from build123d import *

# Parameters (mm, degrees)
BOSS_EXTRU_1_DEPTH = 15


with BuildPart() as part:
    # Esquisse1 → Boss.-Extru.1 (new body)
    with BuildSketch(Plane.XY):
        with BuildLine():
            ThreePointArc((-50, -27.5), (-47.071067812, -34.571067812), (-40, -37.5))
            Line((-40, -37.5), (-35, -37.5))
            Line((-35, -37.5), (-35, -22.5))
            Line((-35, -22.5), (-35, -7.5))
            Line((-35, -7.5), (-25, -7.5))
            Line((-25, -7.5), (-25, -22.5))
            Line((-25, -22.5), (25, -22.5))
            Line((25, -22.5), (25, -7.5))
            Line((25, -7.5), (35, -7.5))
            Line((35, -7.5), (35, -22.5))
            Line((35, -22.5), (35, -37.5))
            Line((35, -37.5), (40, -37.5))
            ThreePointArc((40, -37.5), (47.071067812, -34.571067812), (50, -27.5))
            Line((50, -27.5), (50, 27.5))
            ThreePointArc((50, 27.5), (47.071067812, 34.571067812), (40, 37.5))
            Line((40, 37.5), (7.5, 37.5))
            Line((7.5, 37.5), (7.5, 15))
            Line((7.5, 15), (-7.5, 15))
            Line((-7.5, 15), (-7.5, 37.5))
            Line((-7.5, 37.5), (-40, 37.5))
            ThreePointArc((-40, 37.5), (-47.071067812, 34.571067812), (-50, 27.5))
            Line((-50, 27.5), (-50, -27.5))
        make_face()
    extrude(amount=BOSS_EXTRU_1_DEPTH)


solid = part.part
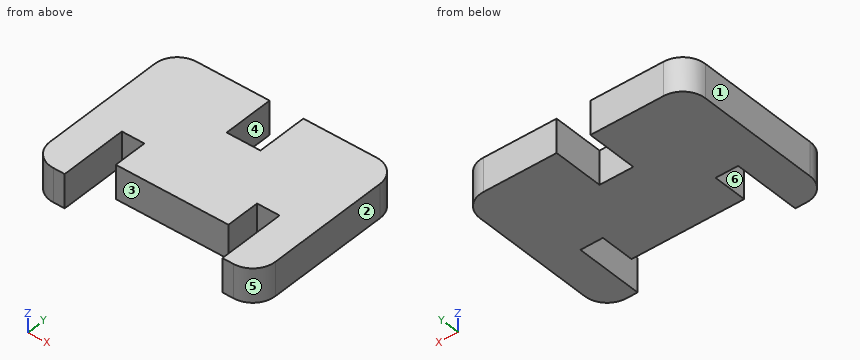
Check sheet for the modelled part. Datum: model origin and axes. Units: mm. Face numbers are marked on the shaded views. A direction names the side the tool comes from. Give positions to 0.01 mm unless a question says otherwise; leave off trailing zeros. Loops run counter-clockwise (first coordinate to the right, second up) from the corner with the lowest first, then second, coordinate; pieces in that order, holes last. Notation, with made-up numbers: M 56,24 L 83,24 A12 ccw 83,42 Z; hole C 47,70 d11. An arc over 180 degrees is marked long. Return JSON: item names as keys, results as strings. Group by question number.
1. Cross-section at D-D on y = -30. Record the boundary of the cut face in (x, z), plus the area to 3 significant figures.
2. Thickness scan on L1, parallel to X at y = -21, z = 3.25; L2, parallel to X at y = 20.5, z = 10.5; L3, parallel to X at y = -25.5, z = 4.75. Record the ranges inside material, lowest first.
3. Tool access check on the marked faces 4, 5 and 6. Record the directions out of +Z, -Z, +X, -X, +Y, -Y that give a thin tool (end or side, any length) a straight path to the whole face; none if there is none.
4. Cross-section at C-C on x = 6. Record the boundary of the cut face in (y, z), plus the area to 4 significant figures.
5. Cross-section at A-A on y = 17.5. Record the boundary of the cut face in (x, z).
6. Cross-section at B-B on z = 1.25. Record the boundary of the cut face in (x, y), plus the area to 3 significant figures.
7. Mould release check, pull along X, two halves, no side actions. Record for the marked faces 1, 2 and 3: released by +X, released by -X, zero draft, split by the parting line, or undercut.
8. Go/stop test with flat-tipped pins: pin 1 (3 mm diameter, centred on x = 14, z = 7, fed in from -Y); pin 2 (2 mm diameter, centred on x = 28, z = 12, fed in from -Y); pin 3 (4 mm diameter, centred on x = -19.5, y = -21.5, fed in from -Z); pin 4 (7.5 mm diameter, centred on y = 31.5, z = 9.5, fed in from -X). Record where each tip stops, or that it passes through.
Return value:
{
 "1": {"outline": "M -49.68,0 L -35,0 L -35,15 L -49.68,15 Z; M 35,0 L 49.68,0 L 49.68,15 L 35,15 Z", "area": "440 mm^2"},
 "2": {"L1": "-50 to -35, -25 to 25, 35 to 50", "L2": "-50 to -7.5, 7.5 to 50", "L3": "-50 to -35, 35 to 50"},
 "3": {"face 4": "+Z, -Z, +Y", "face 5": "+Z, -Z, +X, -Y", "face 6": "+Z, -Z, -Y"},
 "4": {"outline": "M -22.5,0 L 15,0 L 15,15 L -22.5,15 Z", "area": "562.5 mm^2"},
 "5": {"outline": "M -50,0 L -7.5,0 L -7.5,15 L -50,15 Z; M 7.5,0 L 50,0 L 50,15 L 7.5,15 Z"},
 "6": {"outline": "M -50,-27.5 A10 ccw -40,-37.5 L -35,-37.5 L -35,-7.5 L -25,-7.5 L -25,-22.5 L 25,-22.5 L 25,-7.5 L 35,-7.5 L 35,-37.5 L 40,-37.5 A10 ccw 50,-27.5 L 50,27.5 A10 ccw 40,37.5 L 7.5,37.5 L 7.5,15 L -7.5,15 L -7.5,37.5 L -40,37.5 A10 ccw -50,27.5 Z", "area": "5,730 mm^2"},
 "7": {"face 1": "released by -X", "face 2": "released by +X", "face 3": "undercut"},
 "8": {"pin 1": "y = -22.5", "pin 2": "y = -7.5", "pin 3": "z = 0", "pin 4": "x = -50"}
}
